from build123d import *

# Parameters (mm, degrees)
SCHIZZO1_W                   = 550
SCHIZZO1_H                   = 230
ESTRUSIONE_ESTRUSIONE1_DEPTH = 2.5
SCHIZZO2_W                   = 165
SCHIZZO2_H                   = 130
TAGLIO_ESTRUSIONE1_DEPTH     = 10
SCHIZZO3_R                   = 2
TAGLIO_ESTRUSIONE2_DEPTH     = 10


with BuildPart() as part:
    # Schizzo1 → Estrusione-Estrusione1 (new body)
    with BuildSketch(Plane.XY):
        Rectangle(SCHIZZO1_W, SCHIZZO1_H)
    extrude(amount=ESTRUSIONE_ESTRUSIONE1_DEPTH)

    # Schizzo2 → Taglio-Estrusione1 (cut)
    with BuildSketch(Plane(origin=(0, 0, 0), x_dir=(-1, 0, 0), z_dir=(0, 0, -1))):
        with Locations((-192.5, 50)):
            Rectangle(SCHIZZO2_W, SCHIZZO2_H)
    extrude(amount=-TAGLIO_ESTRUSIONE1_DEPTH, mode=Mode.SUBTRACT)

    # Schizzo3 → Taglio-Estrusione2 (cut)
    with BuildSketch(Plane.XY.offset(2.5)):
        with Locations((-83.5, 85)):
            Circle(SCHIZZO3_R)
        with Locations((-257, -100)):
            Circle(SCHIZZO3_R)
        with Locations((257, -100)):
            Circle(SCHIZZO3_R)
    extrude(amount=-TAGLIO_ESTRUSIONE2_DEPTH, mode=Mode.SUBTRACT)


solid = part.part
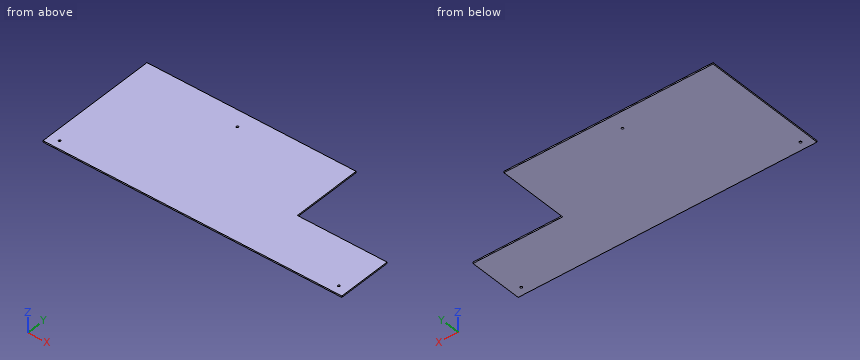
Source: CAD feature listing. Evaluate the final solid. Frame: model axes, mm. Round coordinates to 2 decimals unless told otherwise and drop trailing zeros. Loops run counter-clockwise (first coordinate to the right, second up) from the corner with the lowest first, then second, coordinate; pieces in that order, holes last. Notation, with made-up numbers: (32.25, 32) - (89.25, 32) arc R18 ccw to (89.25, 67) - close; hole circle Ø6 at (-8, -5). An arc over 180 degrees is marked (long way). Write item = value, one per line. Start each with the question number.
(1) Section query B-B, the plane x = 214.5. Output: boundary loops of the cut face in (y, z), plus the area to 3 significant figures.
(2) Section query A-A, the plane z = 1.85. Output: boundary loops of the cut face in (x, y).
(3) Section query C-C, the plane y = 0. Output: boundary loops of the cut face in (x, z).
(4) Ray query, line 1 along Y through (x, z) = (-83.5, 1.55); line 2 along Y through (x, z) = (257, 1); line 3 along Y through (x, z) = (201, 2.2). Return the intervals inside material, ascending. Write a range as from..to.
(5) Pin query (flat end, axial travel): pin 1 (3.5 mm diameter, centred on x = -257, y = -100, fed in from -Z); pin 2 (1.2 mm diameter, centred on y = 28, z = 1, fed in from +X). Return the tip coordinate at first contact, or that it passes through.
Conclusion:
q1.outline = (-115, 0) - (-15, 0) - (-15, 2.5) - (-115, 2.5) - close
q1.area = 250 mm2
q2.outline = (-275, -115) - (275, -115) - (275, -15) - (110, -15) - (110, 115) - (-275, 115) - close; hole circle Ø4 at (-257, -100); hole circle Ø4 at (-83.5, 85); hole circle Ø4 at (257, -100)
q3.outline = (-275, 0) - (110, 0) - (110, 2.5) - (-275, 2.5) - close
q4.line_1 = -115..83, 87..115
q4.line_2 = -115..-102, -98..-15
q4.line_3 = -115..-15
q5.pin_1 = through
q5.pin_2 = 110
